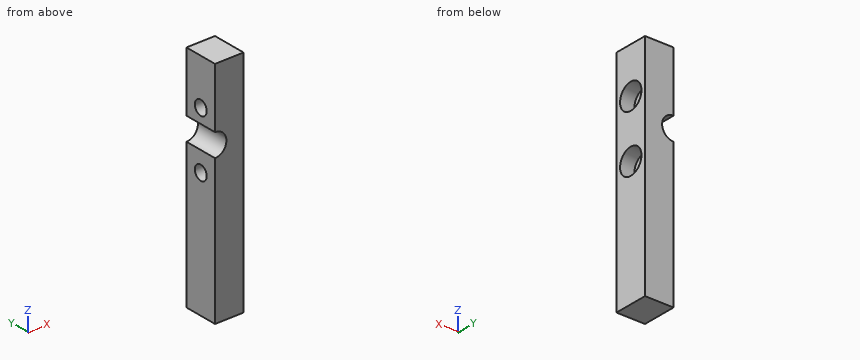
from build123d import *

# Parameters (mm, degrees)
CYLINDER010_R     = 4
CYLINDER010_DEPTH = 12
CYLINDER006_R     = 4.5
CYLINDER006_DEPTH = 5
CYLINDER005_R     = 2.5
CYLINDER005_DEPTH = 5
CYLINDER012_R     = 4.5
CYLINDER012_DEPTH = 5
CYLINDER011_R     = 2.5
CYLINDER011_DEPTH = 5
BOX_W             = 10
BOX_H             = 12
BOX_DEPTH         = 80


with BuildPart() as cylinder010:
    # Cylinder010 → Cylinder010 (new body)
    with BuildSketch(Plane(origin=(32, 12, 55), x_dir=(1, 0, 0), z_dir=(0, -1, 0))):
        Circle(CYLINDER010_R)
    extrude(amount=CYLINDER010_DEPTH)


with BuildPart() as cylinder006:
    # Cylinder006 → Cylinder006 (new body)
    with BuildSketch(Plane(origin=(37, 5, 55), x_dir=(0, 0, -1), z_dir=(1, 0, 0))):
        Circle(CYLINDER006_R)
    extrude(amount=CYLINDER006_DEPTH)


with BuildPart() as obj1:
    # Cylinder005 → Cylinder005 (new body)
    with BuildSketch(Plane(origin=(32, 5, 55), x_dir=(0, 0, -1), z_dir=(1, 0, 0))):
        Circle(CYLINDER005_R)
    extrude(amount=CYLINDER005_DEPTH)

    # Fusion003: union Cylinder006
    add(cylinder006.part)


with BuildPart() as obj1_1:
    # Fusion003 placement: moved
    add(obj1.part.moved(Location((0, 1, 9))))


with BuildPart() as cylinder012:
    # Cylinder012 → Cylinder012 (new body)
    with BuildSketch(Plane(origin=(37, 5, 55), x_dir=(0, 0, -1), z_dir=(1, 0, 0))):
        Circle(CYLINDER012_R)
    extrude(amount=CYLINDER012_DEPTH)


with BuildPart() as screwholes:
    # Cylinder011 → Cylinder011 (new body)
    with BuildSketch(Plane(origin=(32, 5, 55), x_dir=(0, 0, -1), z_dir=(1, 0, 0))):
        Circle(CYLINDER011_R)
    extrude(amount=CYLINDER011_DEPTH)

    # Fusion004: union Cylinder012
    add(cylinder012.part)


with BuildPart() as screwholes_1:
    # Fusion004 placement: moved
    add(screwholes.part.moved(Location((0, 1, -11))))

    # Fusion005: union obj1
    add(obj1_1.part)


with BuildPart() as obj2:
    # Box → Box (new body)
    with BuildSketch(Plane(origin=(32, 0, 0), x_dir=(1, 0, 0), z_dir=(0, 0, 1))):
        with Locations((5, 6)):
            Rectangle(BOX_W, BOX_H)
    extrude(amount=BOX_DEPTH)

    # Cut: cut ScrewHoles
    add(screwholes_1.part, mode=Mode.SUBTRACT)

    # Cut007: cut Cylinder010
    add(cylinder010.part, mode=Mode.SUBTRACT)


solid = obj2.part
Geometry: final body of the model. Coordinates: model frame, mm. Coordinates: 2 decimals unless noted, no trailing zeros. Loops run counter-clockwise (first coordinate to the right, second up) from the corner with the lowest first, then second, coordinate; pieces in that order, holes last. Notation, with made-up numbers: M 12,-1 L 42,-1 A29 cw 42,26 Z; hole C 5,31.25 d5. An arc over 180 degrees is marked long. One line per item, written item: value. Start each with the question number.
1) Material intervals for L1, parallel to Z at x = 39, y = 3; L2, parallel to Z at x = 33.5, y = 6.5; L3, parallel to Z at x = 37.75, y = 3.25, sorted ascending. Write a range as from..to.
2) Pin query (flat end, axial travel): P1, Ø6.5, axis at y = 6, z = 44, coming from the +X side. Return the tip coordinate at first contact, or that it passes through.
3) Cut plane D-D (z = 55). Return loops of the section in (x, y), then the cut area to 3 significant figures.
4) Cut plane C-C (x = 41). Return loops of the section in (y, z), then the cut area to 3 significant figures.
5) Cut plane B-B (z = 44). Return loops of the section in (x, y), then the cut area to 3 significant figures.
6) Cut plane A-A (y = 6). Return loops of the section in (x, z), then the cut area to 3 significant figures.
Evaluation:
1. L1: 0..40.65, 47.35..60.65, 67.35..80
1. L2: 0..41.55, 46.45..51.29, 58.71..61.55, 66.45..80
1. L3: 0..40.44, 47.56..60.44, 67.56..80
2. P1: x = 37
3. outline: M 36,0 L 42,0 L 42,12 L 36,12 Z
3. area: 72.0 mm^2
4. outline: M 0,0 L 12,0 L 12,80 L 0,80 Z; hole C 6,44 d9; hole C 6,64 d9
4. area: 833 mm^2
5. outline: M 32,0 L 42,0 L 42,1.5 L 37,1.5 L 37,3.5 L 32,3.5 Z; M 32,8.5 L 37,8.5 L 37,10.5 L 42,10.5 L 42,12 L 32,12 Z
5. area: 50.0 mm^2
6. outline: M 32,0 L 42,0 L 42,39.5 L 37,39.5 L 37,41.5 L 32,41.5 Z; M 32,46.5 L 37,46.5 L 37,48.5 L 42,48.5 L 42,59.5 L 37,59.5 L 37,61.5 L 32,61.5 L 32,59 A4 cw 32,51 Z; M 32,66.5 L 37,66.5 L 37,68.5 L 42,68.5 L 42,80 L 32,80 Z
6. area: 635 mm^2
